from build123d import *

# Parameters (mm, degrees)
SKETCH4_R           = 82.042
BOSS_EXTRUDE2_DEPTH = 0.79375
SKETCH5_R           = 15.875
CUT_EXTRUDE5_DEPTH  = 117.027624155
CUT_EXTRUDE11_DEPTH = 117.027624155
SKETCH9_R           = 3.175
CUT_EXTRUDE12_DEPTH = 117.027624155
FILLET1_R           = 1.5875
FILLET2_R           = 0.79375


with BuildPart() as part:
    # Sketch4 → Boss-Extrude2 (new body)
    with BuildSketch(Plane.XY):
        Circle(SKETCH4_R)
    extrude(amount=BOSS_EXTRUDE2_DEPTH)

    # Sketch5 → Cut-Extrude5 (cut, through all)
    with BuildSketch(Plane.XY.offset(0.79375)):
        Circle(SKETCH5_R)
    extrude(amount=-CUT_EXTRUDE5_DEPTH, mode=Mode.SUBTRACT)

    # Sketch8 → Cut-Extrude11 (cut, through all)
    with BuildSketch(Plane.XY.offset(0.79375)):
        Polygon((76.869596069, 30.465791131), (75.89758015, 32.812445144), (74.724253144, 32.326437185), (75.696269062, 29.979783172), align=None)
        Polygon((-30.465791131, 76.869596069), (-32.812445144, 75.89758015), (-32.326437185, 74.724253144), (-29.979783172, 75.696269062), align=None)
        Polygon((-75.89758015, 32.812445144), (-76.869596069, 30.465791131), (-75.696269062, 29.979783172), (-74.724253144, 32.326437185), align=None)
        Polygon((-76.869596069, -30.465791131), (-75.89758015, -32.812445144), (-74.724253144, -32.326437185), (-75.696269062, -29.979783172), align=None)
        Polygon((-32.812445144, -75.89758015), (-30.465791131, -76.869596069), (-29.979783172, -75.696269062), (-32.326437185, -74.724253144), align=None)
        Polygon((30.465791131, -76.869596069), (32.812445144, -75.89758015), (32.326437185, -74.724253144), (29.979783172, -75.696269062), align=None)
        Polygon((75.89758015, -32.812445144), (76.869596069, -30.465791131), (75.696269062, -29.979783172), (74.724253144, -32.326437185), align=None)
        Polygon((32.812445144, 75.89758015), (30.465791131, 76.869596069), (29.979783172, 75.696269062), (32.326437185, 74.724253144), align=None)
    extrude(amount=-CUT_EXTRUDE11_DEPTH, mode=Mode.SUBTRACT)

    # Sketch9 → Cut-Extrude12 (cut, through all)
    with BuildSketch(Plane.XY.offset(0.79375)):
        with Locations((22.225, 0)):
            Circle(SKETCH9_R)
        with Locations((36.195, 0)):
            Circle(SKETCH9_R)
        with Locations((61.722, 0)):
            Circle(SKETCH9_R)
        with Locations((75.691993951, 0)):
            Circle(SKETCH9_R)
        with Locations((15.715448212, -15.715448212)):
            Circle(SKETCH9_R)
        with Locations((25.593729945, -25.593729945)):
            Circle(SKETCH9_R)
        with Locations((43.644044748, -43.644044748)):
            Circle(SKETCH9_R)
        with Locations((53.522322204, -53.522322204)):
            Circle(SKETCH9_R)
        with Locations((0, -22.225)):
            Circle(SKETCH9_R)
        with Locations((0, -36.195)):
            Circle(SKETCH9_R)
        with Locations((0, -61.722)):
            Circle(SKETCH9_R)
        with Locations((0, -75.691993951)):
            Circle(SKETCH9_R)
        with Locations((-15.715448212, -15.715448212)):
            Circle(SKETCH9_R)
        with Locations((-25.593729945, -25.593729945)):
            Circle(SKETCH9_R)
        with Locations((-43.644044748, -43.644044748)):
            Circle(SKETCH9_R)
        with Locations((-53.522322204, -53.522322204)):
            Circle(SKETCH9_R)
        with Locations((-22.225, 0)):
            Circle(SKETCH9_R)
        with Locations((-36.195, 0)):
            Circle(SKETCH9_R)
        with Locations((-61.722, 0)):
            Circle(SKETCH9_R)
        with Locations((-75.691993951, 0)):
            Circle(SKETCH9_R)
        with Locations((-15.715448212, 15.715448212)):
            Circle(SKETCH9_R)
        with Locations((-25.593729945, 25.593729945)):
            Circle(SKETCH9_R)
        with Locations((-43.644044748, 43.644044748)):
            Circle(SKETCH9_R)
        with Locations((-53.522322204, 53.522322204)):
            Circle(SKETCH9_R)
        with Locations((0, 22.225)):
            Circle(SKETCH9_R)
        with Locations((0, 36.195)):
            Circle(SKETCH9_R)
        with Locations((0, 61.722)):
            Circle(SKETCH9_R)
        with Locations((0, 75.691993951)):
            Circle(SKETCH9_R)
        with Locations((15.715448212, 15.715448212)):
            Circle(SKETCH9_R)
        with Locations((25.593729945, 25.593729945)):
            Circle(SKETCH9_R)
        with Locations((43.644044748, 43.644044748)):
            Circle(SKETCH9_R)
        with Locations((53.522322204, 53.522322204)):
            Circle(SKETCH9_R)
        with BuildLine():
            Line((21.703545506, 37.329191157), (30.003653075, 45.629298725))
            ThreePointArc((30.003653075, 45.629298725), (20.898342241, 50.45306127), (11.049, 53.480573099))
            Line((11.049, 53.480573099), (11.049, 41.742448407))
            ThreePointArc((11.049, 41.742448407), (16.52427061, 39.893118214), (21.703545506, 37.329191157))
        make_face()
        with BuildLine():
            Line((41.742448407, -11.049), (53.480573099, -11.049))
            ThreePointArc((53.480573099, -11.049), (50.45306127, -20.898342241), (45.629298725, -30.003653075))
            Line((45.629298725, -30.003653075), (37.329191157, -21.703545506))
            ThreePointArc((37.329191157, -21.703545506), (39.893118214, -16.52427061), (41.742448407, -11.049))
        make_face()
        with BuildLine():
            Line((-11.049, -41.742448407), (-11.049, -53.480573099))
            ThreePointArc((-11.049, -53.480573099), (-20.898342241, -50.45306127), (-30.003653075, -45.629298725))
            Line((-30.003653075, -45.629298725), (-21.703545506, -37.329191157))
            ThreePointArc((-21.703545506, -37.329191157), (-16.52427061, -39.893118214), (-11.049, -41.742448407))
        make_face()
        with BuildLine():
            Line((-41.742448407, 11.049), (-53.480573099, 11.049))
            ThreePointArc((-53.480573099, 11.049), (-50.45306127, 20.898342241), (-45.629298725, 30.003653075))
            Line((-45.629298725, 30.003653075), (-37.329191157, 21.703545506))
            ThreePointArc((-37.329191157, 21.703545506), (-39.893118214, 16.52427061), (-41.742448407, 11.049))
        make_face()
    extrude(amount=-CUT_EXTRUDE12_DEPTH, mode=Mode.SUBTRACT)

    # Fillet1
    fillet1_edges = [part.edges().sort_by_distance(p)[0] for p in [
        (21.703545506, 37.329191157, 0.396875),
        (11.049, 41.742448407, 0.396875),
        (11.049, 53.480573099, 0.396875),
        (30.003653075, 45.629298725, 0.396875),
        (37.329191157, -21.703545506, 0.396875),
        (41.742448407, -11.049, 0.396875),
        (53.480573099, -11.049, 0.396875),
        (45.629298725, -30.003653075, 0.396875),
        (-21.703545506, -37.329191157, 0.396875),
        (-11.049, -41.742448407, 0.396875),
        (-11.049, -53.480573099, 0.396875),
        (-30.003653075, -45.629298725, 0.396875),
        (-37.329191157, 21.703545506, 0.396875),
        (-41.742448407, 11.049, 0.396875),
        (-53.480573099, 11.049, 0.396875),
        (-45.629298725, 30.003653075, 0.396875),
    ]]
    fillet(fillet1_edges, radius=FILLET1_R)

    # Fillet2
    # the kernel refuses this fillet: 0.79375 mm, written as the material it adds along each edge
    with BuildSketch(Plane(origin=(-75.696269062, 29.979783172, 0.79375), x_dir=(0.3826834323651269, 0.9238795325112714, 0), z_dir=(0, 0, -1)), Plane(origin=(-32.326437185, 74.724253144, 0.79375), x_dir=(0.9238795325112888, 0.382683432365085, 0), z_dir=(0, 0, -1))) as fillet2_piece_1:
        with BuildLine():
            CenterArc((0.775641503, -0.79375), FILLET2_R, 90, 77.737864874)
            Line((0, -0.62516969), (-0.01551283, -0.621798083))
            ThreePointArc((-0.01551283, -0.621798083), (-0.015875, -0.312584845), (-0.015875, 0))
            Line((-0.015875, 0), (0, 0.015875))
            Line((0, 0.015875), (0.775641503, 0.015875))
            Line((0.775641503, 0.015875), (0.775641503, 0))
        make_face()
    extrude(amount=0.79375)
    with BuildSketch(Plane(origin=(-29.979783172, 75.696269062, 0.79375), x_dir=(-0.3826834323684612, 0.9238795325098903, 0), z_dir=(0, 0, -1)), Plane(origin=(-74.724253144, 32.326437185, 0.79375), x_dir=(-0.9238795325127166, 0.38268343236163754, 0), z_dir=(0, 0, -1))) as fillet2_piece_2:
        with BuildLine():
            CenterArc((0.79375, -0.775641503), FILLET2_R, 102.262135126, 77.737864874)
            Line((0, -0.775641503), (-0.015875, -0.775641503))
            Line((-0.015875, -0.775641503), (-0.015875, 0))
            Line((-0.015875, 0), (0, 0.015875))
            ThreePointArc((0, 0.015875), (0.312584845, 0.015875), (0.621798083, 0.01551283))
            Line((0.621798083, 0.01551283), (0.62516969, 0))
        make_face()
    extrude(amount=0.79375)
    with BuildSketch(Plane(origin=(-74.724253144, -32.326437185, 0.79375), x_dir=(-0.9238795325128379, -0.3826834323613448, 0), z_dir=(0, 0, -1)), Plane(origin=(-29.979783172, -75.696269062, 0.79375), x_dir=(-0.3826834323686382, -0.9238795325098169, 0), z_dir=(0, 0, -1)), Plane(origin=(32.326437185, -74.724253144, 0.79375), x_dir=(0.3826834323615479, -0.9238795325127538, 0), z_dir=(0, 0, -1))) as fillet2_piece_3:
        with BuildLine():
            CenterArc((0.79375, 0.775641503), FILLET2_R, 180, 77.737864874)
            Line((0, 0.775641503), (-0.015875, 0.775641503))
            Line((-0.015875, 0.775641503), (-0.015875, 0))
            Line((-0.015875, 0), (0, -0.015875))
            ThreePointArc((0, -0.015875), (0.312584845, -0.015875), (0.621798083, -0.01551283))
            Line((0.621798083, -0.01551283), (0.62516969, 0))
        make_face()
    extrude(amount=0.79375)
    with BuildSketch(Plane(origin=(-75.696269062, -29.979783172, 0.79375), x_dir=(0.3826834323649975, -0.923879532511325, 0), z_dir=(0, 0, -1)), Plane(origin=(-32.326437185, -74.724253144, 0.79375), x_dir=(0.9238795325112237, -0.38268343236524216, 0), z_dir=(0, 0, -1)), Plane(origin=(29.979783172, -75.696269062, 0.79375), x_dir=(0.9238795325113635, 0.38268343236490476, 0), z_dir=(0, 0, -1))) as fillet2_piece_4:
        with BuildLine():
            CenterArc((0.775641503, 0.79375), FILLET2_R, 192.262135126, 77.737864874)
            Line((0, 0.62516969), (-0.01551283, 0.621798083))
            ThreePointArc((-0.01551283, 0.621798083), (-0.015875, 0.312584845), (-0.015875, 0))
            Line((-0.015875, 0), (0, -0.015875))
            Line((0, -0.015875), (0.775641503, -0.015875))
            Line((0.775641503, -0.015875), (0.775641503, 0))
        make_face()
    extrude(amount=0.79375)
    with BuildSketch(Plane(origin=(75.696269062, -29.979783172, 0.79375), x_dir=(0.9238795325097092, -0.382683432368898, 0), z_dir=(0, 0, -1))) as fillet2_piece_5:
        with BuildLine():
            CenterArc((0.79375, 0.775641503), FILLET2_R, 180, 77.737864875)
            Line((0, 0.775641503), (-0.015875, 0.775641503))
            Line((-0.015875, 0.775641503), (-0.015875, 0))
            Line((-0.015875, 0), (0, -0.015875))
            ThreePointArc((0, -0.015875), (0.312584845, -0.015875), (0.621798084, -0.01551283))
            Line((0.621798084, -0.01551283), (0.62516969, 0))
        make_face()
    extrude(amount=0.79375)
    with BuildSketch(Plane(origin=(74.724253144, -32.326437185, 0.79375), x_dir=(0.38268343236533003, 0.9238795325111873, 0), z_dir=(0, 0, -1))) as fillet2_piece_6:
        with BuildLine():
            CenterArc((0.775641503, 0.79375), FILLET2_R, 192.262135125, 77.737864875)
            Line((0, 0.62516969), (-0.01551283, 0.621798084))
            ThreePointArc((-0.01551283, 0.621798084), (-0.015875, 0.312584845), (-0.015875, 0))
            Line((-0.015875, 0), (0, -0.015875))
            Line((0, -0.015875), (0.775641503, -0.015875))
            Line((0.775641503, -0.015875), (0.775641503, 0))
        make_face()
    extrude(amount=0.79375)
    with BuildSketch(Plane(origin=(75.696269062, 29.979783172, 0.79375), x_dir=(0.9238795325100071, 0.3826834323681794, 0), z_dir=(0, 0, -1)), Plane(origin=(32.326437185, 74.724253144, 0.79375), x_dir=(0.3826834323619378, 0.9238795325125924, 0), z_dir=(0, 0, -1))) as fillet2_piece_7:
        with BuildLine():
            CenterArc((0.79375, -0.775641503), FILLET2_R, 102.262135126, 77.737864875)
            Line((0, -0.775641503), (-0.015875, -0.775641503))
            Line((-0.015875, -0.775641503), (-0.015875, 0))
            Line((-0.015875, 0), (0, 0.015875))
            ThreePointArc((0, 0.015875), (0.312584845, 0.015875), (0.621798084, 0.01551283))
            Line((0.621798084, 0.01551283), (0.62516969, 0))
        make_face()
    extrude(amount=0.79375)
    with BuildSketch(Plane(origin=(74.724253144, 32.326437185, 0.79375), x_dir=(0.3826834323648073, -0.9238795325114039, 0), z_dir=(0, 0, -1)), Plane(origin=(29.979783172, 75.696269062, 0.79375), x_dir=(0.9238795325111434, -0.38268343236543584, 0), z_dir=(0, 0, -1))) as fillet2_piece_8:
        with BuildLine():
            CenterArc((0.775641503, -0.79375), FILLET2_R, 90, 77.737864875)
            Line((0, -0.62516969), (-0.01551283, -0.621798084))
            ThreePointArc((-0.01551283, -0.621798084), (-0.015875, -0.312584845), (-0.015875, 0))
            Line((-0.015875, 0), (0, 0.015875))
            Line((0, 0.015875), (0.775641503, 0.015875))
            Line((0.775641503, 0.015875), (0.775641503, 0))
        make_face()
    extrude(amount=0.79375)


solid = part.part
Here's how the part is built. I have some questions about the finished solid (model axes, mm). Round coordinates to 2 decimals unless told otherwise and drop trailing zeros. Write each loop counter-clockwise with the first axis right and the second up, starting at its lowest first coordinate (ties: lowest second). Pieces come first, ordered by that corner, then holes. Notation, with made-up numbers: (23.5, 5.5) -> (68.5, 5.5) arc R18 cw to (68.5, 24.5) -> close; hole circle Ø10 at (-5, -26.5). An arc over 180 degrees is marked (long way). One line per item, written item: value.
1) I'm going to push a flat-ended pin straight in: pin 1 Ø8.5 at (x, y) = (43.64, 43.64) entering from -Z. Where does the tip first touch, or does it pass through?
Filled sheet:
pin 1: stops at z = 0
2) Suppose I cut it at D-D on y = 69. List the corners of the cut face in (x, z) for me, plus the area to 3 significant figures.
Filled sheet:
outline: (-44.38, 0) -> (44.38, 0) -> (44.38, 0.79) -> (-44.38, 0.79) -> close
area: 70.5 mm2
3) Suppose I cut it at A-A on y = 0. Give the number of separate pieces and of enclosed holes in the cut face, plus the area to 3 significant figures.
Filled sheet:
separate pieces: 10
enclosed holes: 0
area: 64.7 mm2
4) If I drill on line 1 (Y direction, x = -44, z = 0.55); line 2 (Y direction, x = -18, z = 0.05); line 3 (Y direction, x = 20.5, z = 0.2), over which ranges is the centre line in solid material (lowest first)? Write a range as [from, to].
Filled sheet:
line 1: y = [-69.25, -46.8], [-40.49, 11.05], [28.37, 40.49], [46.8, 69.25]
line 2: y = [-80.04, -51.56], [-39.25, -17.92], [-13.51, 13.51], [17.92, 80.04]
line 3: y = [-79.44, -2.67], [2.67, 38], [50.62, 79.44]
5) We'd pull the mould along Y, two halves only. Please class faces 1 (the face through (-57.705, 58.318, 0.391)), 2 (the face through (-58.318, -57.705, 0.391)), 3 (the face through (42.956, -46.744, 0.402)): released by +Y, released by -Y, zero draft, split by the parting line, or undercut.
Filled sheet:
face 1: released by +Y
face 2: released by -Y
face 3: undercut
